Build history of the part. All positions in model axes, mm. Give positions to 0.01 mm unless a question says otherwise; leave off trailing zeros. Loops run counter-clockwise (first coordinate to the right, second up) from the corner with the lowest first, then second, coordinate; pieces in that order, holes last. Notation, with made-up numbers: M -25.5,49 L 26.5,49 A31 cw 26.5,73 Z; hole C 81,33.25 d5. An arc over 180 degrees is marked long. Put each result on its own line as item: value.
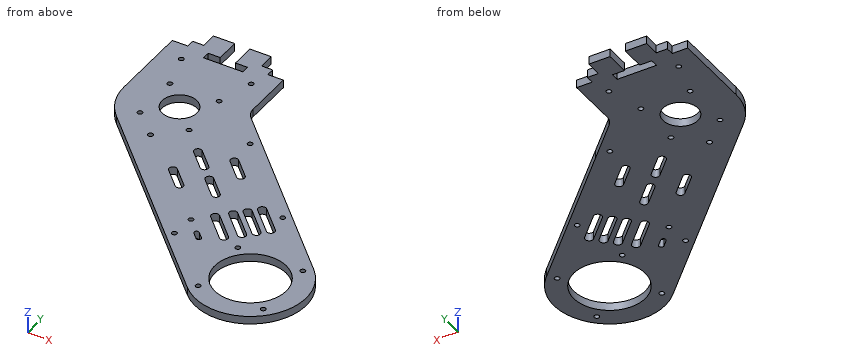
```python
from build123d import *

# Parameters (mm, degrees)
SKETCH1_R           = 1.575
SKETCH1_R_2         = 22.5
SKETCH1_R_3         = 11
BOSS_EXTRUDE1_DEPTH = 5
SKETCH2_W           = 13.4
SKETCH2_H           = 5
BOSS_EXTRUDE2_DEPTH = 5


with BuildPart() as part:
    # Sketch1 → Boss-Extrude1 (new body)
    with BuildSketch(Plane.XY):
        with BuildLine():
            Line((-139.300035894, 89.802561211), (-24.748737342, -24.748737342))
            ThreePointArc((-24.748737342, -24.748737342), (24.748737342, -24.748737342), (24.748737342, 24.748737342))
            Line((24.748737342, 24.748737342), (-54.672802234, 104.170276917))
            Line((-54.672802234, 104.170276917), (-76.622366364, 126.119841047))
            ThreePointArc((-76.622366364, 126.119841047), (-78.790093877, 129.364074535), (-79.551298552, 133.190908859))
            Line((-79.551298552, 133.190908859), (-79.551298552, 164.551298552))
            Line((-79.551298552, 164.551298552), (-89.351298552, 164.551298552))
            Line((-89.351298552, 164.551298552), (-89.351298552, 169.551298552))
            Line((-89.351298552, 169.551298552), (-96.351298552, 169.551298552))
            Line((-96.351298552, 169.551298552), (-96.351298552, 174.551298552))
            Line((-96.351298552, 174.551298552), (-109.751298552, 174.551298552))
            Line((-109.751298552, 174.551298552), (-109.751298552, 169.551298552))
            Line((-109.751298552, 169.551298552), (-109.751298552, 164.551298552))
            Line((-109.751298552, 164.551298552), (-102.201298552, 164.551298552))
            Line((-102.201298552, 164.551298552), (-102.201298552, 159.701298552))
            Line((-102.201298552, 159.701298552), (-126.901298552, 159.701298552))
            Line((-126.901298552, 159.701298552), (-126.901298552, 164.551298552))
            Line((-126.901298552, 164.551298552), (-119.351298552, 164.551298552))
            Line((-119.351298552, 164.551298552), (-119.351298552, 169.551298552))
            Line((-119.351298552, 169.551298552), (-119.351298552, 174.551298552))
            Line((-119.351298552, 174.551298552), (-132.751298552, 174.551298552))
            Line((-132.751298552, 174.551298552), (-132.751298552, 169.551298552))
            Line((-132.751298552, 169.551298552), (-139.751298552, 169.551298552))
            Line((-139.751298552, 169.551298552), (-139.751298552, 164.551298552))
            Line((-139.751298552, 164.551298552), (-149.551298552, 164.551298552))
            Line((-149.551298552, 164.551298552), (-149.551298552, 114.551298552))
            ThreePointArc((-149.551298552, 114.551298552), (-146.88708219, 101.157378419), (-139.300035894, 89.802561211))
        make_face()
        with BuildLine():
            Line((-78.771695424, 51.335952314), (-89.378297142, 61.942554032))
            ThreePointArc((-89.378297142, 61.942554032), (-89.378297142, 65.336666582), (-85.984184592, 65.336666582))
            Line((-85.984184592, 65.336666582), (-75.377582874, 54.730064864))
            ThreePointArc((-75.377582874, 54.730064864), (-75.377582874, 51.335952314), (-78.771695424, 51.335952314))
        make_face(mode=Mode.SUBTRACT)
        with BuildLine():
            ThreePointArc((-68.165093707, 64.770981156), (-68.165093707, 68.165093706), (-64.770981157, 68.165093706))
            Line((-64.770981157, 68.165093706), (-54.164379439, 57.558491989))
            ThreePointArc((-54.164379439, 57.558491989), (-54.164379439, 54.164379439), (-57.558491988, 54.164379439))
            Line((-57.558491988, 54.164379439), (-68.165093707, 64.770981156))
        make_face(mode=Mode.SUBTRACT)
        with Locations((-20.506096654, -20.506096654)):
            Circle(SKETCH1_R, mode=Mode.SUBTRACT)
        with Locations((-56.568542495, 14.142135624)):
            Circle(SKETCH1_R, mode=Mode.SUBTRACT)
        with Locations((20.506096654, -20.506096654)):
            Circle(SKETCH1_R, mode=Mode.SUBTRACT)
        Circle(SKETCH1_R_2, mode=Mode.SUBTRACT)
        with Locations((-55.401816306, 29.450997436)):
            Circle(SKETCH1_R, mode=Mode.SUBTRACT)
        with BuildLine():
            ThreePointArc((-47.623641713, 19.5515025), (-47.623641713, 21.672822843), (-45.502321369, 21.672822843))
            Line((-45.502321369, 21.672822843), (-41.966787463, 18.137288937))
            ThreePointArc((-41.966787463, 18.137288937), (-41.966787463, 16.015968594), (-44.088107807, 16.015968594))
            Line((-44.088107807, 16.015968594), (-47.623641713, 19.5515025))
        make_face(mode=Mode.SUBTRACT)
        with BuildLine():
            ThreePointArc((-47.72970773, 37.123106012), (-47.72970773, 40.658639918), (-44.194173824, 40.658639918))
            Line((-44.194173824, 40.658639918), (-30.0520382, 26.516504294))
            ThreePointArc((-30.0520382, 26.516504294), (-30.0520382, 22.980970389), (-33.587572106, 22.980970389))
            Line((-33.587572106, 22.980970389), (-47.72970773, 37.123106012))
        make_face(mode=Mode.SUBTRACT)
        with Locations((-20.506096654, 20.506096654)):
            Circle(SKETCH1_R, mode=Mode.SUBTRACT)
        with BuildLine():
            ThreePointArc((-40.658639918, 44.194173824), (-40.658639918, 47.72970773), (-37.123106012, 47.72970773))
            Line((-37.123106012, 47.72970773), (-22.980970389, 33.587572106))
            ThreePointArc((-22.980970389, 33.587572106), (-22.980970389, 30.0520382), (-26.516504294, 30.0520382))
            Line((-26.516504294, 30.0520382), (-40.658639918, 44.194173824))
        make_face(mode=Mode.SUBTRACT)
        with BuildLine():
            ThreePointArc((-35.001785669, 49.851028074), (-35.001785669, 53.38656198), (-31.466251763, 53.38656198))
            Line((-31.466251763, 53.38656198), (-17.324116139, 39.244426356))
            ThreePointArc((-17.324116139, 39.244426356), (-17.324116139, 35.70889245), (-20.859650045, 35.70889245))
            Line((-20.859650045, 35.70889245), (-35.001785669, 49.851028074))
        make_face(mode=Mode.SUBTRACT)
        with BuildLine():
            ThreePointArc((-29.344931419, 55.507882323), (-29.344931419, 59.043416229), (-25.809397513, 59.043416229))
            Line((-25.809397513, 59.043416229), (-11.66726189, 44.901280605))
            ThreePointArc((-11.66726189, 44.901280605), (-11.66726189, 41.365746699), (-15.202795796, 41.365746699))
            Line((-15.202795796, 41.365746699), (-29.344931419, 55.507882323))
        make_face(mode=Mode.SUBTRACT)
        with Locations((-14.142135624, 56.568542495)):
            Circle(SKETCH1_R, mode=Mode.SUBTRACT)
        with Locations((20.506096654, 20.506096654)):
            Circle(SKETCH1_R, mode=Mode.SUBTRACT)
        with Locations((-114.551298552, 84.551298552)):
            Circle(SKETCH1_R, mode=Mode.SUBTRACT)
        with Locations((-130.051298552, 99.051298552)):
            Circle(SKETCH1_R, mode=Mode.SUBTRACT)
        with Locations((-114.551298552, 114.551298552)):
            Circle(SKETCH1_R_3, mode=Mode.SUBTRACT)
        with BuildLine():
            ThreePointArc((-86.549870017, 83.155757468), (-86.549870017, 86.549870017), (-83.155757468, 86.549870017))
            Line((-83.155757468, 86.549870017), (-72.54915575, 75.943268299))
            ThreePointArc((-72.54915575, 75.943268299), (-72.54915575, 72.54915575), (-75.943268299, 72.54915575))
            Line((-75.943268299, 72.54915575), (-86.549870017, 83.155757468))
        make_face(mode=Mode.SUBTRACT)
        with BuildLine():
            ThreePointArc((-65.336666582, 85.984184592), (-65.336666582, 89.378297142), (-61.942554032, 89.378297142))
            Line((-61.942554032, 89.378297142), (-51.335952314, 78.771695424))
            ThreePointArc((-51.335952314, 78.771695424), (-51.335952314, 75.377582874), (-54.730064864, 75.377582874))
            Line((-54.730064864, 75.377582874), (-65.336666582, 85.984184592))
        make_face(mode=Mode.SUBTRACT)
        with Locations((-99.051298552, 99.051298552)):
            Circle(SKETCH1_R, mode=Mode.SUBTRACT)
        with Locations((-64.396887007, 105.308740477)):
            Circle(SKETCH1_R, mode=Mode.SUBTRACT)
        with Locations((-130.051298552, 130.051298552)):
            Circle(SKETCH1_R, mode=Mode.SUBTRACT)
        with Locations((-136.551298552, 152.551298552)):
            Circle(SKETCH1_R, mode=Mode.SUBTRACT)
        with Locations((-99.051298552, 130.051298552)):
            Circle(SKETCH1_R, mode=Mode.SUBTRACT)
        with Locations((-92.551298552, 152.551298552)):
            Circle(SKETCH1_R, mode=Mode.SUBTRACT)
    extrude(amount=-BOSS_EXTRUDE1_DEPTH)

    # Sketch2 → Boss-Extrude2 (add)
    with BuildSketch(Plane.XY):
        with Locations((-126.051298552, 177.051298552)):
            Rectangle(SKETCH2_W, SKETCH2_H)
        with Locations((-103.051298552, 177.051298552)):
            Rectangle(SKETCH2_W, SKETCH2_H)
    extrude(amount=-BOSS_EXTRUDE2_DEPTH)


solid = part.part
```
Q1. Slice it at C-C (z = -1). State how many separate pieces and enclosed holes the cut face has, and give its area (3 significant figures).
Here are the results:
separate pieces: 1
enclosed holes: 26
area: 14,100 mm²
Q2. Slice it at B-B (x = 0). List the corners of the cut face in (y, z).
Here are the results:
outline: M -35,-5 L -22.5,-5 L -22.5,0 L -35,0 Z; M 22.5,-5 L 49.5,-5 L 49.5,0 L 22.5,0 Z
Q3. Slice it at A-A (y = 0). List the corners of the cut face in (x, z).
Here are the results:
outline: M -49.5,-5 L -22.5,-5 L -22.5,0 L -49.5,0 Z; M 22.5,-5 L 35,-5 L 35,0 L 22.5,0 Z
Q4. Probe line 1 (X direction, y = 81.5, z = -3.9); line 2 (X direction, y = 31.5, z = -2.6); line 3 (Y direction, x = -86.5, z = -1). List the from-to ranges inside material, lowest first. Write a range as from..to.
Here are the results:
line 1: -131..-84.89, -78.11..-60.85, -54.06..-32
line 2: -81..-42.11, -35.04..-27.96, -22.27..18
line 3: 37..59.06, 65.73..83.11, 86.6..164.55
Q5. Drop flat-ended pins along their axis: pin 1 Ø2.5 at (y, z) = (168, -2.5) entering from -X; pin 2 Ø2 at (y, z) = (11.5, -2.5) entering from -X; pin 3 Ø1 at (x, z) = (-20, -3) entering from -Y; pin 4 Ø3 at (x, y) = (-14.14, 56.57) entering from +Z. Give the stop position or say it passes through.
Here are the results:
pin 1: x = -139.75
pin 2: x = -62
pin 3: y = -29.06
pin 4: through
